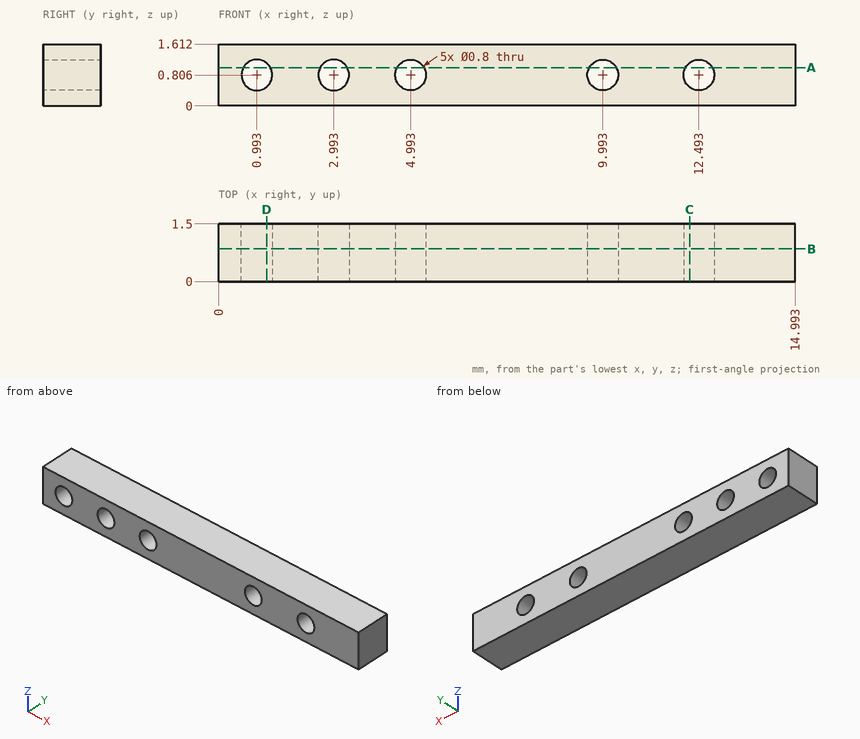
Here's the drawing with two shaded views (mm, measured from the low corner). I have some questions. Give positions to 0.01 mm unless a question says otherwise; leave off trailing zeros. Order: outer loops, then holes, each group sorted by start corner. A loop starts at its lowest first (then second) coordinate and runs counter-clockwise, first axis right, second up.
Q1. Suppose I cut it at C-C, the plane x = 12.25. Write out the boundary of the cut face in (y, z) (1 decimal).
Q2. If I drill on line 1 along X through (y, z) = (1, 0.85) (1 decimal); line 2 along Z through (x, y) = (10, 0.3); line 3 along X through (y, z) = (0.8, 1), over which ranges is the centre line in solid material (lowest first)?
Q3. Suppose I cut it at A-A, the plane z = 1. Write out the boundary of the cut face in (x, y).
Q4. Suppose I cut it at B-B, the plane y = 0.85. Write out the boundary of the cut face in (x, z).
Q5. Suppose I cut it at D-D, the plane x = 1.25. Write out the boundary of the cut face in (y, z).
Solution:
1. outline: (0, 0) - (1.5, 0) - (1.5, 0.5) - (0, 0.5) - close; (0, 1.1) - (1.5, 1.1) - (1.5, 1.6) - (0, 1.6) - close
2. line 1: x = 0 to 0.6, 1.4 to 2.6, 3.4 to 4.6, 5.4 to 9.6, 10.4 to 12.1, 12.9 to 15
2. line 2: z = 0 to 0.41, 1.21 to 1.61
2. line 3: x = 0 to 0.64, 1.34 to 2.64, 3.34 to 4.64, 5.34 to 9.64, 10.34 to 12.14, 12.84 to 14.99
3. outline: (0, 0) - (0.64, 0) - (0.64, 1.5) - (0, 1.5) - close; (1.34, 0) - (2.64, 0) - (2.64, 1.5) - (1.34, 1.5) - close; (3.34, 0) - (4.64, 0) - (4.64, 1.5) - (3.34, 1.5) - close; (5.34, 0) - (9.64, 0) - (9.64, 1.5) - (5.34, 1.5) - close; (10.34, 0) - (12.14, 0) - (12.14, 1.5) - (10.34, 1.5) - close; (12.84, 0) - (14.99, 0) - (14.99, 1.5) - (12.84, 1.5) - close
4. outline: (0, 0) - (14.99, 0) - (14.99, 1.61) - (0, 1.61) - close; hole circle Ø0.8 at (0.99, 0.81); hole circle Ø0.8 at (2.99, 0.81); hole circle Ø0.8 at (4.99, 0.81); hole circle Ø0.8 at (9.99, 0.81); hole circle Ø0.8 at (12.49, 0.81)
5. outline: (0, 0) - (1.5, 0) - (1.5, 0.5) - (0, 0.5) - close; (0, 1.11) - (1.5, 1.11) - (1.5, 1.61) - (0, 1.61) - close
